```python
from build123d import *

# Parameters (mm, degrees)
EXTRUDE_1_DEPTH      = 10
EXTRUDE_2_DEPTH      = 5
EXTRUDE_2_DEPTH_BACK = 32.5
SKETCH_2_R           = 4.5
SKETCH_2_R_2         = 2.5
DRAFT_1_ANGLE        = 3
DRAFT_2_ANGLE        = 3
EXTRUDE_3_DEPTH      = 3
EXTRUDE_3_DEPTH_BACK = 3


with BuildPart() as part:
    # 草图1 → 凸台-拉伸1 (new body)
    with BuildSketch(Plane.XY):
        Polygon((0, 38.5), (4, 42.5), (23.5, 42.5), (27.5, 38.5), (27.5, 4), (23.5, 0), (4, 0), (0, 4), align=None)
    extrude(amount=EXTRUDE_1_DEPTH)

    # 草图2 → 凸台-拉伸2 (add, two sides: drawn at the far end of the back side and taken through both)
    with BuildSketch(Plane.ZY.offset(-EXTRUDE_2_DEPTH_BACK)):
        with Locations((5, 10.5)):
            Circle(SKETCH_2_R)
        with Locations((5, 10.5)):
            Circle(SKETCH_2_R_2, mode=Mode.SUBTRACT)
    extrude(amount=EXTRUDE_2_DEPTH + EXTRUDE_2_DEPTH_BACK)

    # 拔模1
    draft_1_faces = [part.faces().sort_by_distance(p)[0] for p in [
        (30, 10.5, 0.5),
    ]]
    draft(draft_1_faces, Plane(origin=(27.5, 4, 10), x_dir=(0, 0, 1), z_dir=(1, 0, 0)), DRAFT_1_ANGLE)

    # 拔模2
    draft_2_faces = [part.faces().sort_by_distance(p)[0] for p in [
        (-2.5, 10.5, 0.5),
    ]]
    draft(draft_2_faces, Plane(origin=(0, 4, 10), x_dir=(0, 0, -1), z_dir=(-1, 0, 0)), DRAFT_2_ANGLE)

    # 草图3 → 凸台-拉伸3 (add, two sides: drawn at the far end of the back side and taken through both)
    with BuildSketch(Plane.XY.offset(5).offset(-EXTRUDE_3_DEPTH_BACK)):
        with BuildLine():
            Line((31, 34.5), (25.5, 34.5))
            Line((25.5, 34.5), (25.5, 22.5))
            Line((25.5, 22.5), (31, 22.5))
            ThreePointArc((31, 22.5), (37, 28.5), (31, 34.5))
        make_face()
        with BuildLine():
            Line((31, 32.5), (27.5, 32.5))
            Line((27.5, 32.5), (27.5, 24.5))
            Line((27.5, 24.5), (31, 24.5))
            ThreePointArc((31, 24.5), (35, 28.5), (31, 32.5))
        make_face(mode=Mode.SUBTRACT)
    extrude(amount=EXTRUDE_3_DEPTH + EXTRUDE_3_DEPTH_BACK)


solid = part.part
```
Input: part model. Units: mm. Frame: model coordinates. A direction names the side the tool comes from. Give positions to 0.01 mm unless a question says otherwise; leave off trailing zeros. Order: outer loops, then holes, each group sorted by start corner. A loop starts at its lowest first (then second) coordinate and runs counter-clockwise, first axis right, second up. Notation, with made-up numbers: (-5.5, 59) - (26.5, 59) arc R22 ccw to (26.5, 66) - close; hole circle Ø1 at (-36, -31). An arc over 180 degrees is marked (long way). Put each result on its own line as item: value.
Item 1: Section query D-D, the plane x = 24. Return loops of the section in (y, z).
Found:
outline: (0.5, 0) - (42, 0) - (42, 10) - (0.5, 10) - close
Item 2: Ray query, L1, parallel to Y at x = 32, z = 4.5; L2, parallel to Y at x = 31.55, z = 5; L3, parallel to Y at x = -0.5, z = 4.5. Return the intervals inside material, ascending. Write a range as from..to.
Found:
L1: y = 6.27..8.05, 12.95..14.73, 22.58..24.63, 32.37..34.42
L2: y = 6.21..8, 13..14.79, 22.53..24.54, 32.46..34.47
L3: y = 6.05..8.05, 12.95..14.95
Item 3: Section query A-A, the plane y = 28.5. Return loops of the section in (x, z), then the cut area to 3 significant figures.
Found:
outline: (0, 0) - (27.5, 0) - (27.5, 10) - (0, 10) - close; (35, 2) - (37, 2) - (37, 8) - (35, 8) - close
area: 287 mm^2
Item 4: Contact query for flat-ended pins moving along their axis: pin 1 (1 mm diameter, centred on x = 28.5, z = 5, fed in from +Y); pin 2 (5 mm diameter, centred on x = 32.5, y = 8, fed in from +Z); pin 3 (3 mm diameter, centred on y = 21.5, z = 4.5, fed in from -X). Output: stop coordinate, or through.
Found:
pin 1: stops at y = 34.5
pin 2: stops at z = 9.29
pin 3: stops at x = 0
Item 5: Section query C-C, the plane y = 10.5. Return loops of the section in (x, z).
Found:
outline: (-5, 0.76) - (0, 0.5) - (0, 0) - (27.5, 0) - (27.5, 0.5) - (32.5, 0.76) - (32.5, 2.5) - (27.5, 2.5) - (27.5, 7.5) - (32.5, 7.5) - (32.5, 9.24) - (27.5, 9.5) - (27.5, 10) - (0, 10) - (0, 9.5) - (-5, 9.24) - (-5, 7.5) - (0, 7.5) - (0, 2.5) - (-5, 2.5) - close
Item 6: Draft query along X for faces 6 (the flat face through (25, 41, 5)), 7 (the flat face through (14, 42.5, 5)), 8 (the flat face through (-5, 7.7, 4.9)), 9 (the flat face through (27.5, 25, 5)). Return one class per face: +X half, -X half, draft (parallel to the pull), parting line (faces both ways), or undercut.
Found:
face 6: +X half
face 7: draft
face 8: -X half
face 9: undercut
Item 7: Access query for faces 1 (the cylindrical face through (-2.47, 8.28, 6.15)), 2 (the flat face through (29, 24.5, 5)), 3 (the flat face through (29, 34.5, 5)), 4 (the flat face through (35.4, 28.6, 2)), 5 (the flat face through (32.5, 7.7, 4.9)). Directions: +Z, -Z, +X, -X, +Y, -Y. A direction counts if a zero-diameter tool reaches every point of the face in a straight line with its end or side. Return the directions, or none.
Found:
face 1: -X
face 2: +Z, -Z
face 3: +Z, -Z, +X, +Y
face 4: -Z, +X, +Y
face 5: +Z, -Z, +X, -Y
